from build123d import *

# Parameters (mm, degrees)
F0_W      = 50
F0_H      = 50
F1_DEPTH  = 50
F2_W      = 30
F2_H      = 30
F3_DEPTH  = 25
F4_W      = 10
F4_H      = 10
F5_DEPTH  = 20
F6_W      = 10
F6_H      = 10
F7_DEPTH  = 20
F8_W      = 10
F8_H      = 10
F9_DEPTH  = 15
F10_W     = 5
F10_H     = 5
F11_DEPTH = 3


with BuildPart() as f1:
    # F0 (on Top) → F1 (new body)
    with BuildSketch(Plane.XY):
        with Locations((-25, 25)):
            Rectangle(F0_W, F0_H)
    extrude(amount=F1_DEPTH)

    # F2 (on face) → F3 (join)
    with BuildSketch(Plane.XY.offset(50)):
        with Locations((-25, 25)):
            Rectangle(F2_W, F2_H)
    extrude(amount=F3_DEPTH)

    # F4 (on face) → F5 (join)
    with BuildSketch(Plane.XZ):
        with Locations((-25, 25)):
            Rectangle(F4_W, F4_H)
    extrude(amount=F5_DEPTH)

    # F6 (on face) → F7 (join)
    with BuildSketch(Plane(origin=(0, 50, 0), x_dir=(-1, 0, 0), z_dir=(0, 1, 0))):
        with Locations((25, 25)):
            Rectangle(F6_W, F6_H)
    extrude(amount=F7_DEPTH)

    # F8 (on face) → F9 (join)
    with BuildSketch(Plane(origin=(0, 0, 0), x_dir=(1, 0, 0), z_dir=(0, 0, -1))):
        with Locations((-23.593899, -35)):
            Rectangle(F8_W, F8_H)
        with Locations((-23.962104, -15)):
            Rectangle(F8_W, F8_H)
    extrude(amount=F9_DEPTH)

    # F10 (on face) → F11 (join)
    with BuildSketch(Plane.YZ.offset(-10)):
        with Locations((17.5, 67.5)):
            Rectangle(F10_W, F10_H)
        with Locations((32.5, 67.5)):
            Rectangle(F10_W, F10_H)
    extrude(amount=F11_DEPTH)


solid = f1.part
Input: part model. Units: mm. Frame: model coordinates. A direction names the side the tool comes from. Give positions to 0.01 mm unless a question says otherwise; leave off trailing zeros. Loops run counter-clockwise (first coordinate to the right, second up) from the corner with the lowest first, then second, coordinate; pieces in that order, holes last. Notation, with made-up numbers: M 18,11 L 39,11 A19 cw 39,41 Z; hole C 76,55 d4. An arc over 180 degrees is marked long. Use one line per item in the form item = value.
1. Section query C-C, the plane y = 12.5. Return the cut outline in (x, z), and give its area (3 significant figures).
Numbers:
outline = M -50,0 L -28.96,0 L -28.96,-15 L -18.96,-15 L -18.96,0 L 0,0 L 0,50 L -10,50 L -10,75 L -40,75 L -40,50 L -50,50 Z
area = 3,400 mm²
2. Line query: L1, parallel to Z at x = -24.5, y = 56; L2, parallel to Y at x = -40, z = 22; L3, parallel to X at y = 22, z = 59. Output: solid intervals per line, ascending.
Numbers:
L1 = 20 to 30
L2 = 0 to 50
L3 = -40 to -10
3. Pull-direction query (Y, two-part tool) for faces 6 (the face through (-25, 9, 50)), 7 (the face through (-25, -20, 25)), 8 (the face through (-24, 20, -7)), 9 (the face through (-25, 70, 25)); classes: released by +Y, released by -Y, zero draft, split by the parting line, or undercut.
Numbers:
face_6 = zero draft
face_7 = released by -Y
face_8 = undercut
face_9 = released by +Y
4. First-contact query: pin 1 (5 mm diameter, centred on x = -8, z = 49.5, fed in from +Y); pin 2 (8 mm diameter, centred on y = 14.5, z = -4.5, fed in from +X); pin 3 (1.5 mm diameter, centred on x = -8, y = 32, fed in from +Z). Flat tips, straight axial feed; report the tip coordinate or a pass-through.
Numbers:
pin_1 = 50
pin_2 = -18.96
pin_3 = 70
5. Section query A-A, the plane z = -10. Return the cut outline in (x, y), and give its area (3 significant figures).
Numbers:
outline = M -28.96,10 L -18.96,10 L -18.96,20 L -28.96,20 Z; M -28.59,30 L -18.59,30 L -18.59,40 L -28.59,40 Z
area = 200 mm²
6. Section query D-D, the plane y = 27. Return the cut outline in (x, z), and give its area (3 significant figures).
Numbers:
outline = M -50,0 L 0,0 L 0,50 L -10,50 L -10,75 L -40,75 L -40,50 L -50,50 Z
area = 3,250 mm²
7. Reachability of faces 1 (the face through (-24, 30, -7)), 2 (the face through (-9, 20, 67)), 3 (the face through (-25, 10, 62)), 4 (the face through (-25, 40, 62)), 5 (the face through (-28.594, 35, -7)) from +Z, -Z, +X, -X, +Y, -Y: full face, straight path, thin tool, end or side. Return the list, or none.
Numbers:
face_1 = -Z, +X, -X
face_2 = +Z, +X
face_3 = +Z, +X, -X, -Y
face_4 = +Z, +X, -X, +Y
face_5 = -Z, -X, +Y
8. Section query B-B, the plane x = -22.5. Return the cut outline in (y, z).
Numbers:
outline = M -20,20 L 0,20 L 0,0 L 10,0 L 10,-15 L 20,-15 L 20,0 L 30,0 L 30,-15 L 40,-15 L 40,0 L 50,0 L 50,20 L 70,20 L 70,30 L 50,30 L 50,50 L 40,50 L 40,75 L 10,75 L 10,50 L 0,50 L 0,30 L -20,30 Z
